```python
from build123d import *

# Parameters (mm, degrees)
SKETCH6_W          = 90
SKETCH6_H          = 12
SKETCH7_R          = 8.5
SKETCH7_R_2        = 2.5
CUT_EXTRUDE1_DEPTH = 340
SKETCH8_R          = 2.5
CUT_EXTRUDE2_DEPTH = 8


with BuildPart() as part:
    # Sweep2: sweep along a path in Sketch4
    with BuildLine(Plane.XY) as sweep2_path:
        Line((-65, 350), (-65, 10))
        ThreePointArc((-65, 10), (-62.071067812, 2.928932188), (-55, 0))
        Line((-55, 0), (55, 0))
        ThreePointArc((55, 0), (62.071067812, 2.928932188), (65, 10))
        Line((65, 10), (65, 350))
        Line((65, 350), (-65, 350))
    # Sketch6 → Sweep2 (sweep)
    with BuildSketch(Plane(origin=(0, 0, 0), x_dir=(0, 0, -1), z_dir=(1, 0, 0))):
        with Locations((0, 350)):
            Rectangle(SKETCH6_W, SKETCH6_H)
    sweep(path=sweep2_path.line, transition=Transition.RIGHT)

    # Sketch7 → Cut-Extrude1 (cut)
    with BuildSketch(Plane(origin=(0, 356, 0), x_dir=(1, 0, 0), z_dir=(0, 1, 0))):
        with Locations((60, 0)):
            Circle(SKETCH7_R)
        with Locations((-60, 0)):
            Circle(SKETCH7_R)
        with Locations((-47, -37)):
            Circle(SKETCH7_R_2)
        with Locations((-47, 37)):
            Circle(SKETCH7_R_2)
        with Locations((47, -37)):
            Circle(SKETCH7_R_2)
        with Locations((47, 37)):
            Circle(SKETCH7_R_2)
    extrude(amount=-CUT_EXTRUDE1_DEPTH, mode=Mode.SUBTRACT)

    # Sketch8 → Cut-Extrude2 (cut)
    with BuildSketch(Plane(origin=(0, 6, 0), x_dir=(1, 0, 0), z_dir=(0, 1, 0))):
        with Locations((47, 37)):
            Circle(SKETCH8_R)
        with Locations((-47, 37)):
            Circle(SKETCH8_R)
        with Locations((-47, -37)):
            Circle(SKETCH8_R)
        with Locations((47, -37)):
            Circle(SKETCH8_R)
    extrude(amount=-CUT_EXTRUDE2_DEPTH, mode=Mode.SUBTRACT)


solid = part.part
```
Build history of the part. All positions in model axes, mm. A direction names the side the tool comes from. Give positions to 0.01 mm unless a question says otherwise; leave off trailing zeros. Loops run counter-clockwise (first coordinate to the right, second up) from the corner with the lowest first, then second, coordinate; pieces in that order, holes last. Notation, with made-up numbers: (-3.75, 84) - (3.25, 84) arc R7 ccw to (3.25, 93) - close; hole circle Ø3 at (47, -2). An arc over 180 degrees is marked (long way). Use a Markdown table: item, result.
(1) Which spindle directions (+Z, -Z, +X, -X, +Y, -Y) get a long thin tool onto all of the face, cutting with end or side? Do faces 4 (the face through (68.11, 188.38, -2.55)), 5 (the face through (59, 179, -9)), 6 (the face through (-1, 356, -1)). Say none if no direction does.
Taken from the geometry:
| item | result |
|---|---|
| face 4 | +Y |
| face 5 | +Z, -Z |
| face 6 | +Z, -Z, +X, -X, +Y |
(2) Pull direction Z, two halves, no side cores. Call faces 1 (the face through (-68.49, 188.38, -0.37)), 2 (the face through (63, 174, -45)), 3 (the face through (-66.437, -1.189, 0.63)): +Z half, -Z half, draft (parallel to the pull), parting line (faces both ways), or undercut.
Taken from the geometry:
| item | result |
|---|---|
| face 1 | undercut |
| face 2 | -Z half |
| face 3 | draft |
(3) Drop flat-ended pins along their axis: pin 1 Ø7.5 at (x, z) = (62.5, 1.5) entering from +Y; pin 2 Ø4 at (x, z) = (47, -37) entering from +Y. Give the stop position or say it passes through.
Taken from the geometry:
| item | result |
|---|---|
| pin 1 | y = 16 |
| pin 2 | y = -2 |
(4) Wall check: line 1 along Z through (x, y) = (-47, 347); line 2 along X through (y, z) = (350, 37); line 3 along X through (y, z) = (222, -25). Give the ranges that are in metal, low to high.
Taken from the geometry:
| item | result |
|---|---|
| line 1 | -45 to -39.5, -34.5 to 34.5, 39.5 to 45 |
| line 2 | -71 to -49.5, -44.5 to 44.5, 49.5 to 71 |
| line 3 | -71 to -59, 59 to 71 |
(5) Band-saw the part on A-A (z = 12.5). Give the cut face in (x, y).
Taken from the geometry:
| item | result |
|---|---|
| outline | (-71, 10) arc R16 ccw to (-55, -6) - (55, -6) arc R16 ccw to (71, 10) - (71, 356) - (-71, 356) - close; hole (-59, 10) arc R4 ccw to (-55, 6) - (55, 6) arc R4 ccw to (59, 10) - (59, 344) - (-59, 344) - close |
(6) Band-saw the part on B-B (x = 0.5). Give the cut face in (y, z), and give its area (3 significant figures).
Taken from the geometry:
| item | result |
|---|---|
| outline | (-6, -45) - (6, -45) - (6, 45) - (-6, 45) - close; (344, -45) - (356, -45) - (356, 45) - (344, 45) - close |
| area | 2,160 mm2 |
(7) Band-saw the part on C-C (y = 105). Give the cut face in (x, z), and give its area (3 significant figures).
Taken from the geometry:
| item | result |
|---|---|
| outline | (-71, -45) - (-59, -45) - (-59, -8.44) arc R8.5 cw (long way) to (-59, 8.44) - (-59, 45) - (-71, 45) - close; (59, -45) - (71, -45) - (71, 45) - (59, 45) - (59, 8.44) arc R8.5 cw (long way) to (59, -8.44) - close |
| area | 1,900 mm2 |
